Can you work these out from the model? Positions are in its coordinate system, mm. A direction names the side the tool comes from. Give positions to 0.01 mm unless a question says otherwise; leave off trailing zeros. Order: outer loops, then holes, each group sorted by start corner. A loop starts at its lowest first (then second) coordinate and runs counter-clockwise, first axis right, second up. Notation, with made-up numbers: (73.5, 24.25) -> (78.5, 24.25) arc R35 ccw to (78.5, 59.25) -> close; hole circle Ø2 at (1.5, 65). An arc over 180 degrees is marked (long way). Answer as CSV lines item,"result".
```python
from build123d import *

# Parameters (mm, degrees)
SKETCH1_R           = 47
SKETCH1_R_2         = 43
BOSS_EXTRUDE1_DEPTH = 1.5
CUT_EXTRUDE1_DEPTH  = 67.484960705


with BuildPart() as part:
    # Sketch1 → Boss-Extrude1 (new, symmetric)
    with BuildSketch(Plane.XY):
        Circle(SKETCH1_R)
        Circle(SKETCH1_R_2, mode=Mode.SUBTRACT)
    extrude(amount=BOSS_EXTRUDE1_DEPTH, both=True)

    # Sketch2 → Cut-Extrude1 (cut, through all)
    with BuildSketch(Plane(origin=(0, 0, 0), x_dir=(0, 0, -1), z_dir=(1, 0, 0))):
        Polygon((-7.723456939, 6.371672693), (7.049357633, -7.110313422), (7.723456939, -6.371672693), (-7.049357633, 7.110313422), align=None)
    extrude(amount=-CUT_EXTRUDE1_DEPTH, mode=Mode.SUBTRACT)


solid = part.part
```
Item 1: Imagine slicing it at A-A, the plane x = 0. Please give me the cut outline in (y, z).
Numbers:
outline,"(-47, -1.5) -> (-43, -1.5) -> (-43, 1.5) -> (-47, 1.5) -> close; (43, -1.5) -> (47, -1.5) -> (47, 1.5) -> (43, 1.5) -> close"
Item 2: Imagine slicing it at B-B, the plane y = -5. Please give me the cut outline in (x, z).
Numbers:
outline,"(-46.73, -1.5) -> (-42.71, -1.5) -> (-42.71, 1.5) -> (-46.73, 1.5) -> close; (42.71, -1.5) -> (46.73, -1.5) -> (46.73, 1.5) -> (42.71, 1.5) -> close"
Item 3: We'd pull the mould along Y, two halves only. Please class faces 3 (the flat face through (21, -38, 1.5)), 4 (the flat face through (-44.95, 0.66, -0.02)): released by +Y, released by -Y, zero draft, split by the parting line, or undercut.
Numbers:
face 3,"zero draft"
face 4,"undercut"
Item 4: Imagine slicing it at C-C, the plane z = 0.3. Please give me the cut outline in (x, y).
Numbers:
outline,"(-47, -0.4) arc R47 ccw (long way) to (-46.99, 0.95) -> (-42.99, 0.95) arc R43 cw (long way) to (-43, -0.4) -> close"
Item 5: For pin 1 (1 mm diameter, centred on x = -11.5, z = 0.5, fed in from +Y); pin 2 (1.5 mm diameter, centred on x = 16.5, z = 0, fed in from -Y), each with a flat end and sliding along its axis, tell me the tip position at first contact or that it passes through.
Numbers:
pin 1,"stops at y = 45.69"
pin 2,"stops at y = -44.28"
Item 6: For faces 1 (the flat face through (21, -38, -1.5)), 2 (the flat face through (-44.95, -0.66, 0.02)), which set-ups out of +Z, -Z, +X, -X, +Y, -Y let a thin tool reach every point of the face, with its end or its side?
Numbers:
face 1,"-Z, +X, -X, +Y, -Y"
face 2,"-X"
Item 7: Please list where these lines run through material, in increasing order: line 1 along X through (y, z) = (17, 1); line 2 along X through (y, z) = (23.5, -0.75); line 3 along Y through (x, z) = (15.5, 0.65).
Numbers:
line 1,"x = -43.82 to -39.5, 39.5 to 43.82"
line 2,"x = -40.7 to -36.01, 36.01 to 40.7"
line 3,"y = -44.37 to -40.11, 40.11 to 44.37"
